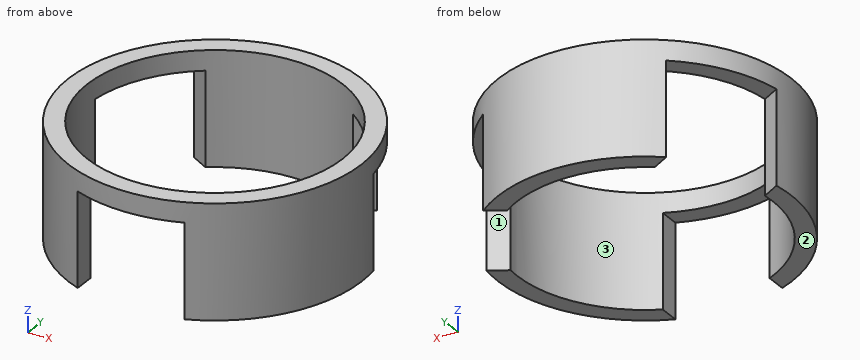
```python
from build123d import *

# Parameters (mm, degrees)
F0_R      = 15.5
F0_R_2    = 13.5
F1_DEPTH  = 10
F3_R      = 15.5
F3_R_2    = 13.5
F4_DEPTH  = 2
F5_W      = 11.3
F5_H      = 18.3407559019
F6_DEPTH  = 9.9
F7_COUNT  = 3
F9_R      = 8
F10_DEPTH = 25


# Not quite as in the source:
# - the program builds the solid bodies; features that only make, move or delete a surface that nothing else refers to are left out


with BuildPart() as f1:
    # F0 (on Top) → F1 (new body)
    with BuildSketch(Plane.XY):
        Circle(F0_R)
        Circle(F0_R_2, mode=Mode.SUBTRACT)
    extrude(amount=F1_DEPTH)

    # F3 (on offset) → F4 (join)
    with BuildSketch(Plane.XY.offset(10)):
        Circle(F3_R)
        Circle(F3_R_2, mode=Mode.SUBTRACT)
    extrude(amount=F4_DEPTH)

    # F5 (on Top) → F6 (cut)
    with BuildSketch(Plane.XY):
        with Locations((-1.81e-07, -13.0000018069)):
            Rectangle(F5_W, F5_H)
    f6 = extrude(amount=F6_DEPTH, mode=Mode.SUBTRACT)

    # F7: F6 ×3 about axis
    f7_axis = Axis((0, 0, 0), (0, 0, -1))
    for i in range(1, F7_COUNT):
        add(f6.rotate(f7_axis, i * 360 / F7_COUNT), mode=Mode.SUBTRACT)

    # F9 (on offset) → F10 (cut)
    with BuildSketch(Plane.XY.offset(22)):
        Circle(F9_R)
    extrude(amount=-F10_DEPTH, mode=Mode.SUBTRACT)


solid = f1.part
```
Work out the finished part from the listing and answer in its coordinate system (mm). Face numbers are marked on the shaded views. Round coordinates to 2 decimals unless told otherwise and drop trailing zeros. Write each loop counter-clockwise with the first axis right and the second up, starting at its lowest first coordinate (ties: lowest second). Pieces come first, ordered by that corner, then holes. Notation, with made-up numbers: (15, 80) - (65, 80) arc R13 cw to (65, 88) - close; hole circle Ø8 at (10, 65.25). An arc over 180 degrees is marked (long way). Return JSON: item names as keys, results as strings. Group by question number.
Q1. The part is cut by section D-D on z = 10.5. Write down the section's boundary in (x, y), then the cut area to 3 significant figures.
Q2. Find the intervals of material crossed by L1, parallel to X at y = 0, z = 8.75; L2, parallel to X at y = -2, z = 7.25; L3, parallel to Y at x = 0, z = 7.75, in increasing order.
Q3. The part is cut by section A-A on x = 0. Write down the section's boundary in (y, z).
Q4. The part is cut by section C-C on z = 8.5. Write down the section's boundary in (x, y).
Q5. The part is cut by section B-B on y = 0. Write down the section's boundary in (x, z), then the cut area to 3 significant figures.
Q6. The mould has two halves that part along Y. Classify the marked faces 1, 2 and 3: released by +Y, released by -Y, zero draft, split by the parting line, or undercut.
Q7. Each of these flat-tipped pins is pushed along its axis until it touches: pin 1 Ø2 at (x, z) = (3.5, 5.5) entering from -Y; pin 2 Ø3 at (y, z) = (-12, 8) entering from -X; pin 3 Ø1.7 at (y, z) = (-14, 6.5) entering from -X. Where does it stop, or does it pass through?
Solved:
{
 "1": {"outline": "circle Ø31 at (0, 0); hole circle Ø27 at (0, 0)", "area": "182 mm²"},
 "2": {"L1": "-15.5 to -13.5, 13.5 to 15.5", "L2": "-15.37 to -13.35, 13.35 to 15.37", "L3": "13.5 to 15.5"},
 "3": {"outline": "(-15.5, 9.9) - (-13.5, 9.9) - (-13.5, 12) - (-15.5, 12) - close; (13.5, 0) - (15.5, 0) - (15.5, 12) - (13.5, 12) - close"},
 "4": {"outline": "(-15.32, 2.32) arc R15.5 ccw to (-5.65, -14.43) - (-5.65, -12.26) arc R13.5 cw to (-13.44, 1.24) - close; (-9.67, 12.11) - (-7.79, 11.02) arc R13.5 cw to (7.79, 11.02) - (9.67, 12.11) arc R15.5 ccw to start; (5.65, -14.43) arc R15.5 ccw to (15.32, 2.32) - (13.44, 1.24) arc R13.5 cw to (5.65, -12.26) - close"},
 "5": {"outline": "(-15.5, 0) - (-13.5, 0) - (-13.5, 12) - (-15.5, 12) - close; (13.5, 0) - (15.5, 0) - (15.5, 12) - (13.5, 12) - close", "area": "48.0 mm²"},
 "6": {"face 1": "released by +Y", "face 2": "zero draft", "face 3": "undercut"},
 "7": {"pin 1": "y = 12.73", "pin 2": "x = -11.4", "pin 3": "x = -8.21"}
}
